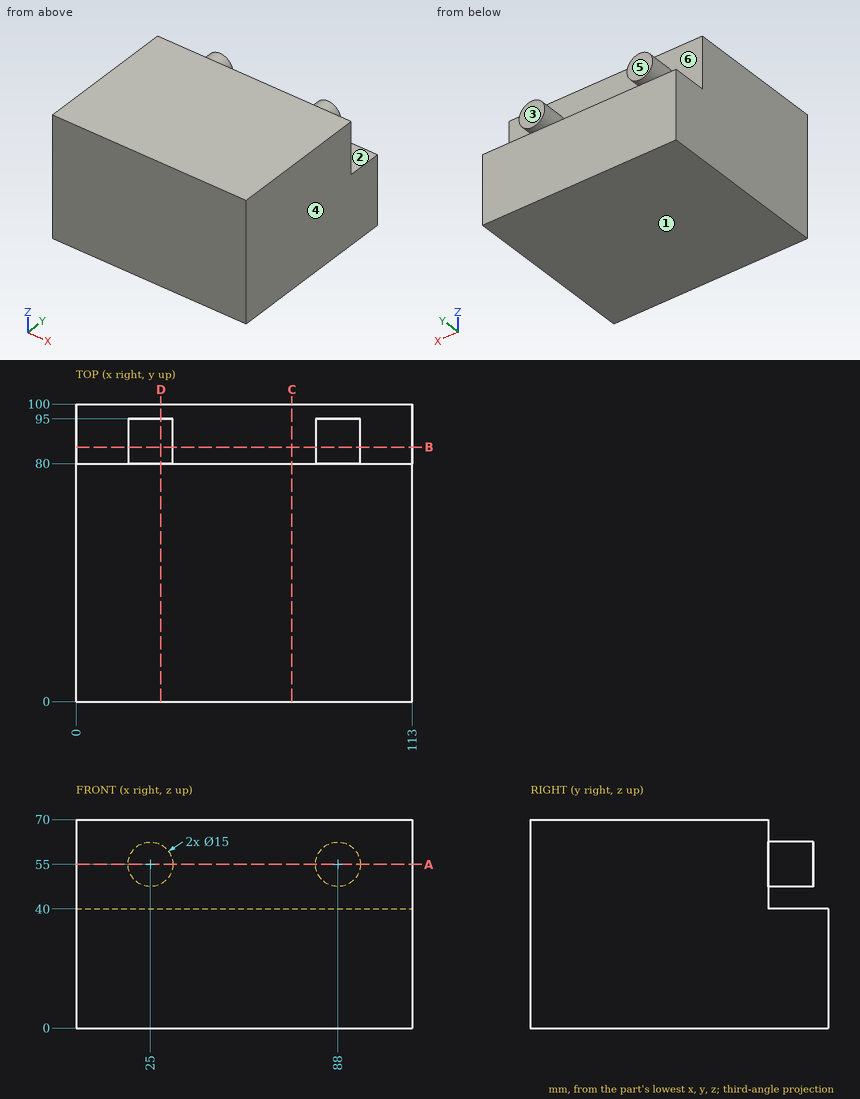
Check sheet for the drawn part. Datum: minimum x, y, z corner. Units: mm. A direction names the side the tool comes from. Give positions to 0.01 mm unless a question says otherwise; leave off trailing zeros. Order: outer loops, then holes, each group sorted by start corner. A loop starts at its lowest first (then second) coordinate and runs counter-clockwise, first axis right, second up.
1. Draft check along Z on the marked faces 1, 2 and 3. Enter one of: pulls with the +Z half, pulls with the -Z half, needs draft (parallel to the pull), parting line crosses it, or undercut.
Completed:
face 1: pulls with the -Z half
face 2: undercut
face 3: needs draft
2. Sectioned sample at C-C (x = 72.5). Record the boundary of the cut face in (y, z).
Completed:
outline: (0, 0) - (100, 0) - (100, 40) - (80, 40) - (80, 70) - (0, 70) - close
3. Depth check by flat-ended pin: pin 1 (10 mm diameter, centred on x = 40, y = 88.5, fed in from +Z); pin 2 (24 mm diameter, centred on x = 61, z = 57, fed in from +Y); pin 3 (12 mm diameter, centred on x = 86, z = 55, fed in from +Y). Enter the tip coordinate at first touch or a pass-through.
Completed:
pin 1: stops at z = 40
pin 2: stops at y = 80
pin 3: stops at y = 95
4. Sectioned sample at A-A (z = 55). Record the boundary of the cut face in (x, y).
Completed:
outline: (0, 0) - (113, 0) - (113, 80) - (95.5, 80) - (95.5, 95) - (80.5, 95) - (80.5, 80) - (32.5, 80) - (32.5, 95) - (17.5, 95) - (17.5, 80) - (0, 80) - close
5. Sectioned sample at D-D (x = 28.5). Record the boundary of the cut face in (y, z).
Completed:
outline: (0, 0) - (100, 0) - (100, 40) - (80, 40) - (80, 48.37) - (95, 48.37) - (95, 61.63) - (80, 61.63) - (80, 70) - (0, 70) - close
6. Scan lines: line 1 (Z direction, x = 93, y = 88); line 2 (Y direction, x = 33, z = 64); line 3 (Z direction, x = 106, y = 95.5). Record each from-to range of solid material in increasing order.
Completed:
line 1: z = 0 to 40, 49.41 to 60.59
line 2: y = 0 to 80
line 3: z = 0 to 40
7. Access from +Z, -Z, +X, -X, +Y, -Y to the whole of each face (thin tool, end or side, straight path). Record for the marked faces 4, 5 and 6.
Completed:
face 4: +Z, -Z, +X, +Y, -Y
face 5: +Z, +X, -X, +Y
face 6: +Y
8. Sectioned sample at B-B (y = 85.5). Record the boundary of the cut face in (x, z).
Completed:
outline: (0, 0) - (113, 0) - (113, 40) - (0, 40) - close; circle Ø15 at (25, 55); circle Ø15 at (88, 55)
